Work out the finished part from the listing and answer in its coordinate system (mm). A direction names the side the tool comes from. Round coordinates to 2 decimals unless told otherwise and drop trailing zeros. Order: outer loops, then holes, each group sorted by start corner. A loop starts at its lowest first (then second) coordinate and runs counter-clockwise, first axis right, second up. Notation, with made-up numbers: (71.25, -24.75) -> (93.25, -24.75) arc R11 cw to (93.25, -19.75) -> close; hole circle Ø7 at (21, 70). An arc over 180 degrees is marked (long way). Use one line per item in the form item = value.
```python
from build123d import *

# Parameters (mm, degrees)
BOSS_EXTRUDE1_START = -6
SKETCH1_W           = 22
SKETCH1_H           = 32
BOSS_EXTRUDE1_DEPTH = 12
BOSS_EXTRUDE2_START = -4
SKETCH2_W           = 18
SKETCH2_H           = 28
BOSS_EXTRUDE2_DEPTH = 11


with BuildPart() as part:
    # Sketch1 → Boss-Extrude1 (new body)
    with BuildSketch(Plane.XY.offset(BOSS_EXTRUDE1_START)):
        with Locations((0, 16)):
            Rectangle(SKETCH1_W, SKETCH1_H)
    extrude(amount=BOSS_EXTRUDE1_DEPTH)


with BuildPart() as body_2:
    # Sketch2 → Boss-Extrude2 (new body)
    with BuildSketch(Plane.XY.offset(BOSS_EXTRUDE2_START)):
        with Locations((0, 16)):
            Rectangle(SKETCH2_W, SKETCH2_H)
    extrude(amount=BOSS_EXTRUDE2_DEPTH)


with BuildPart() as part_1:
    add(part.part)

    # Combine1: cut body 2
    add(body_2.part, mode=Mode.SUBTRACT)


solid = part_1.part
```
Item 1: The part is cut by section B-B, the plane y = 19. Give the vertices of the cut face in (x, z).
Findings:
outline = (-11, -6) -> (11, -6) -> (11, 6) -> (9, 6) -> (9, -4) -> (-9, -4) -> (-9, 6) -> (-11, 6) -> close
Item 2: For faces 1 (the flat face through (-9, 16, 1)), 2 (the flat face through (0, 16, -6)), determine the directions among +Z, -Z, +X, -X, +Y, -Y from which every point of the face is accessible in a straight line to the end or side of a thin tool.
Findings:
face_1 = +Z
face_2 = -Z, +X, -X, +Y, -Y
Item 3: A flat-ended cylindrical pin translates along its axis: P1, Ø8, axis at x = 0.5, y = 22, coming from the +Z side. Find the tip coordinate at first contact, or state that the pin passes through.
Findings:
P1 = -4
Item 4: The part is cut by section C-C, the plane x = -3.5. Give the vertices of the cut face in (y, z).
Findings:
outline = (0, -6) -> (32, -6) -> (32, 6) -> (30, 6) -> (30, -4) -> (2, -4) -> (2, 6) -> (0, 6) -> close
Item 5: Consider line 1 along Y through (x, z) = (-0.25, -3.75); line 2 along X through (y, z) = (24, 3.25); line 3 along Z through (x, y) = (7, 15.5). Determine where each line is inside the solid, lowest interval first.
Findings:
line_1 = 0 to 2, 30 to 32
line_2 = -11 to -9, 9 to 11
line_3 = -6 to -4
Item 6: Determine the mould class of faces 3 (the flat face through (0, 0, 0)), 4 (the flat face through (-11, 16, 0)), 5 (the flat face through (0, 30, 1)), 6 (the flat face through (0, 2, 1)) for opening direction X: released by +X, released by -X, zero draft, split by the parting line, or undercut.
Findings:
face_3 = zero draft
face_4 = released by -X
face_5 = undercut
face_6 = undercut
Item 7: The part is cut by section A-A, the plane z = 5.25. Give the vertices of the cut face in (x, y).
Findings:
outline = (-11, 0) -> (11, 0) -> (11, 32) -> (-11, 32) -> close; hole (-9, 2) -> (9, 2) -> (9, 30) -> (-9, 30) -> close
